```python
from build123d import *

# Parameters (mm, degrees)
BOX003_W               = 6.5
BOX003_H               = 4.8
BOX003_DEPTH           = 8
CYLINDER003_R          = 2.5
CYLINDER003_DEPTH      = 7.5
CYLINDER002_R          = 4
CYLINDER002_DEPTH      = 40
CYLINDER002_ROLL_ANGLE = 90
BOX_W                  = 8
BOX_H                  = 40
BOX_DEPTH              = 7
CYLINDER001_R          = 2.5
CYLINDER001_DEPTH      = 39
CYLINDER001_ROLL_ANGLE = 90
CYLINDER_R             = 4
CYLINDER_DEPTH         = 40
CYLINDER_ROLL_ANGLE    = 90
BOX004_W               = 10
BOX004_H               = 40
BOX004_DEPTH           = 2
BOX002_W               = 10
BOX002_H               = 40
BOX002_DEPTH           = 2


with BuildPart() as cube:
    # Box003 → Box003 (new body)
    with BuildSketch(Plane(origin=(-0.25, 0, 0), x_dir=(1, 0, 0), z_dir=(0, 0, 1))):
        with Locations((3.25, 2.4)):
            Rectangle(BOX003_W, BOX003_H)
    extrude(amount=BOX003_DEPTH)


with BuildPart() as rx_module:
    # Cylinder003 → Cylinder003 (new body)
    with BuildSketch(Plane(origin=(3, 1, 0), x_dir=(1, 0, 0), z_dir=(0, 0, 1))):
        Circle(CYLINDER003_R)
    extrude(amount=CYLINDER003_DEPTH)

    # Fusion001: union Cube
    add(cube.part)


with BuildPart() as rx_module_1:
    # Fusion001 placement: moved
    add(rx_module.part.moved(Location((25, 39, 4))))


with BuildPart() as base_cut:
    # Cylinder002 → Cylinder002 (new body)
    with BuildSketch(Plane.XY):
        Circle(CYLINDER002_R)
    extrude(amount=CYLINDER002_DEPTH)


with BuildPart() as base_cut_1:
    # Cylinder002 roll: moved
    add(base_cut.part.rotate(Axis((0, 0, 0), (1, 0, 0)), CYLINDER002_ROLL_ANGLE))


with BuildPart() as base_cut_2:
    # Cylinder002 placement: moved
    add(base_cut_1.part.moved(Location((28, 45, 11))))


with BuildPart() as cut:
    # Box → Box (new body)
    with BuildSketch(Plane(origin=(24, 5, 4), x_dir=(1, 0, 0), z_dir=(0, 0, 1))):
        with Locations((4, 20)):
            Rectangle(BOX_W, BOX_H)
    extrude(amount=BOX_DEPTH)

    # Cut: cut Base_cut
    add(base_cut_2.part, mode=Mode.SUBTRACT)


with BuildPart() as cylinder001:
    # Cylinder001 → Cylinder001 (new body)
    with BuildSketch(Plane.XY):
        Circle(CYLINDER001_R)
    extrude(amount=CYLINDER001_DEPTH)


with BuildPart() as cylinder001_1:
    # Cylinder001 roll: moved
    add(cylinder001.part.rotate(Axis((0, 0, 0), (1, 0, 0)), CYLINDER001_ROLL_ANGLE))


with BuildPart() as cylinder001_2:
    # Cylinder001 placement: moved
    add(cylinder001_1.part.moved(Location((28, 44, 9.5))))


with BuildPart() as cut002:
    # Cylinder → Cylinder (new body)
    with BuildSketch(Plane.XY):
        Circle(CYLINDER_R)
    extrude(amount=CYLINDER_DEPTH)


with BuildPart() as cut002_1:
    # Cylinder roll: moved
    add(cut002.part.rotate(Axis((0, 0, 0), (1, 0, 0)), CYLINDER_ROLL_ANGLE))


with BuildPart() as cut002_2:
    # Cylinder placement: moved
    add(cut002_1.part.moved(Location((28, 45, 11))))

    # Cut001: cut Cylinder001
    add(cylinder001_2.part, mode=Mode.SUBTRACT)

    # Fusion: union Cut
    add(cut.part)

    # Cut002: cut Rx Module
    add(rx_module_1.part, mode=Mode.SUBTRACT)


with BuildPart() as pcb001:
    # Box004 → Box004 (new body)
    with BuildSketch(Plane(origin=(14, 5, 4), x_dir=(1, 0, 0), z_dir=(0, 0, 1))):
        with Locations((5, 20)):
            Rectangle(BOX004_W, BOX004_H)
    extrude(amount=BOX004_DEPTH)


with BuildPart() as fusion002:
    # Box002 → Box002 (new body)
    with BuildSketch(Plane(origin=(32, 5, 4), x_dir=(1, 0, 0), z_dir=(0, 0, 1))):
        with Locations((5, 20)):
            Rectangle(BOX002_W, BOX002_H)
    extrude(amount=BOX002_DEPTH)

    # Fusion002: union Cut002, PCB001
    add(cut002_2.part)
    add(pcb001.part)


solid = fusion002.part
```
Geometry check sheet. Reference: the model listing, model coordinates, mm. A direction names the side the tool comes from. Coordinates: 2 decimals unless noted, no trailing zeros. Order: outer loops, then holes, each group sorted by start corner. A loop starts at its lowest first (then second) coordinate and runs counter-clockwise, first axis right, second up.
Q1. Sectioned sample at B-B on z = 9. Record the cut outline in (x, y).
Reply:
outline: (24, 5) - (25.55, 5) - (25.55, 39) - (24.75, 39) - (24.75, 43.8) - (25.55, 43.8) - (25.55, 44) - (30.45, 44) - (30.45, 43.8) - (31.25, 43.8) - (31.25, 39) - (30.45, 39) - (30.45, 5) - (32, 5) - (32, 45) - (24, 45) - close
Q2. Tool access check on faces 1 (the face through (28, 44, 10)), 2 (the face through (19, 25, 6)), 3 (the face through (25.87, 38.69, 11.22)), 4 (the face through (14, 25, 5)). Record the directions out of +Z, -Z, +X, -X, +Y, -Y that give a thin tool (end or side, any length) a straight path to the whole face; none if there is none.
Reply:
face 1: -Y
face 2: +Z, -X, +Y, -Y
face 3: -Z
face 4: +Z, -Z, -X, +Y, -Y
Q3. Draft check along X on faces 5 (the face through (24, 25, 8)), 6 (the face through (32, 25, 8)), 7 (the face through (37, 25, 6)), 8 (the face through (27.46, 22.24, 7.06)). Enter one of: released by +X, released by -X, zero draft, split by the parting line, or undercut.
Reply:
face 5: released by -X
face 6: released by +X
face 7: zero draft
face 8: undercut
Q4. Thickness scan on probe 1 along X at (y, z) = (42.5, 10); probe 2 along X at (y, z) = (43.95, 9.5); probe 3 along Y at (x, z) = (29.5, 9). Record the ranges inside material, lowest first.
Reply:
probe 1: x = 24 to 24.75, 31.25 to 32
probe 2: x = 24 to 25.5, 30.5 to 32
probe 3: y = 44 to 45
Q5. Sectioned sample at A-A on y = 32. Record the cut outline in (x, z), and give its area (3 significant figures).
Reply:
outline: (14, 4) - (42, 4) - (42, 6) - (32, 6) - (32, 11) arc R4 ccw to (24, 11) - (24, 6) - (14, 6) - close; hole circle Ø5 at (28, 9.5)
area: 101 mm2
Q6. Sectioned sample at C-C on x = 21. Record the cut outline in (y, z).
Reply:
outline: (5, 4) - (45, 4) - (45, 6) - (5, 6) - close
Q7. Sectioned sample at D-D on z = 12.5. Record the cut outline in (x, y), and give its area (3 significant figures).
Reply:
outline: (24.29, 5) - (31.71, 5) - (31.71, 45) - (24.29, 45) - close
area: 297 mm2
Q8. Depth check by flat-ended pin: pin 1 Ø3 at (x, y) = (39, 17.5) entering from +Z; pin 2 Ø6 at (y, z) = (22.5, 12.5) entering from -X; pin 3 Ø1.5 at (y, z) = (31, 12.5) entering from -X. Enter the tip coordinate at first touch or a pass-through.
Reply:
pin 1: stops at z = 6
pin 2: stops at x = 24
pin 3: stops at x = 24.07
